Read the model definition and answer for the solid it produces. Units are mm, in the model's axes. A direction names the side the tool comes from. Coordinates: 2 decimals unless noted, no trailing zeros. Order: outer loops, then holes, each group sorted by start corner. A loop starts at its lowest first (then second) coordinate and runs counter-clockwise, first axis right, second up. Notation, with made-up numbers: (68, 5) - (95, 5) arc R17 ccw to (95, 24) - close; hole circle Ø5 at (89.25, 88.25). An arc over 180 degrees is marked (long way). Answer as a JSON object with one key per item and string values. Group by question number.
from build123d import *

# Parameters (mm, degrees)
F2_R     = 0.5
F2_R_2   = 0.75
F6_W     = 0.5
F6_H     = 0.575756
F8_R     = 0.254
F9_R     = 0.254
F10_SIZE = 0.508


with BuildPart() as f1:
    # F0 (on Front) → F1 (revolve)
    with BuildSketch(Plane.XZ):
        Polygon((0, 5), (0, 3), (5.08, 3), (5.08, 0), (29.92, 0), (29.92, 3), (35, 3), (35, 6), (12, 6), (12, 5), align=None)
    revolve(axis=Axis((17.5, 0, 0), (-1, 0, 0)))

    # F4: sweep along a path in F3
    with BuildLine(Plane.XZ) as f4_path:
        ThreePointArc((37.670611, -1.684892), (33.885817, -0.426085), (29.92, 0))
    # F2 (on face) → F4 (sweep)
    with BuildSketch(Plane.YZ.offset(29.92)):
        with BuildLine():
            ThreePointArc((2, 0), (1.5, 0.5), (1, 0))
            ThreePointArc((1, 0), (1.5, -0.5), (2, 0))
        make_face()
        with BuildLine():
            ThreePointArc((2.25, 0), (1.5, 0.75), (0.75, 0))
            ThreePointArc((0.75, 0), (1.5, -0.75), (2.25, 0))
        make_face()
        with BuildLine():
            ThreePointArc((2, 0), (1.5, -0.5), (1, 0))
            ThreePointArc((1, 0), (1.5, 0.5), (2, 0))
        make_face(mode=Mode.SUBTRACT)
        with Locations((-1.5, 0)):
            Circle(F2_R)
        with Locations((-1.5, 0)):
            Circle(F2_R_2)
        with Locations((-1.5, 0)):
            Circle(F2_R, mode=Mode.SUBTRACT)
    sweep(path=f4_path.line)

    # F5: sweep along a path in F3
    with BuildLine(Plane.XZ) as f5_path:
        ThreePointArc((29.92, 0), (35.652775, -0.901979), (40.831604, -3.52076))
    # F2 (on face) → F5 (sweep)
    with BuildSketch(Plane.YZ.offset(29.92)):
        with Locations((-1.5, 0)):
            Circle(F2_R)
        with BuildLine():
            ThreePointArc((2, 0), (1.5, 0.5), (1, 0))
            ThreePointArc((1, 0), (1.5, -0.5), (2, 0))
        make_face()
    sweep(path=f5_path.line)

    # F6 (on Top) → F7 (revolve, cut)
    with BuildSketch(Plane.XY):
        with Locations((32.466017, -5.805497)):
            Rectangle(F6_W, F6_H)
    revolve(axis=Axis((32.14075, 0, 0), (-1, 0, 0)), mode=Mode.SUBTRACT)

    # F8
    f8_edges = [f1.edges().sort_by_distance(p)[0] for p in [
        (12, 0, -5),
    ]]
    fillet(f8_edges, radius=F8_R)

    # F9
    f9_edges = [f1.edges().sort_by_distance(p)[0] for p in [
        (0, 0, -5),
    ]]
    fillet(f9_edges, radius=F9_R)

    # F10
    f10_edges = [f1.edges().sort_by_distance(p)[0] for p in [
        (0, 0, -3),
    ]]
    chamfer(f10_edges, length=F10_SIZE)


solid = f1.part
1. A cutting plane is placed at C-C on x = 21. Write down the section's boundary in (y, z).
2. For faces 4 (the flat face through (29.92, 0, 0)), 5 (the flat face through (5.08, 0, 0)), 6 (the cylindrical face through (22, 0, -6)), determine the directions among +Z, -Z, +X, -X, +Y, -Y from which every point of the face is accessible in a straight line to the end or side of a thin tool.
3. A cutting plane is placed at B-B on x = 8.5. Write down the section's boundary in (y, z), and give its area (3 significant figures).
4. Given pin 1 (5 mm diameter, centred on x = 22, z = 3.5, fed in from -Y); pin 2 (6.5 mm diameter, centred on y = 0, z = 0.5, fed in from +X); pin 3 (3 mm diameter, centred on x = 15, y = -3.5, fed in from +Z), each flat-ended and moving along its own axis, determine where each tip first touches the part or whether it passes through.
5. For a pull along Z with two mould halves and no side action, classify faces 1 (the flat face through (32.716, -3, -5)), 2 (the flat face through (40.828, 1.493, -3.526)), 3 (the cylindrical face through (3, 0, -3)) as pulls with the +Z half, pulls with the -Z half, needs draft (parallel to the pull), parting line crosses it, or undercut.
6. Straight lines are drawn through the part: L1, parallel to X at y = -4.5, z = 0.25; L2, parallel to X at y = -3.5, z = 4.5; L3, parallel to X at y = -2.5, z = 4.75. For each, find the intervals that lie inside material, in ascending order.
Derived:
{
 "1": {"outline": "circle Ø12 at (0, 0)"},
 "2": {"face 4": "none", "face 5": "-X", "face 6": "+X, -X"},
 "3": {"outline": "circle Ø10 at (0, 0)", "area": "78.5 mm2"},
 "4": {"pin 1": "stops at y = -5.92", "pin 2": "stops at x = 40.11", "pin 3": "stops at z = 5.66"},
 "5": {"face 1": "needs draft", "face 2": "pulls with the -Z half", "face 3": "undercut"},
 "6": {"L1": "x = 0 to 35", "L2": "x = 12 to 32.22, 32.72 to 35", "L3": "x = 12 to 35"}
}
